from build123d import *

# Parameters (mm, degrees)
F2_SIZE = 1.5
F3_SIZE = 0.5


with BuildPart() as f1:
    # F0 (on Right) → F1 (revolve)
    with BuildSketch(Plane.YZ):
        Polygon((-3.7, 0), (-2, 0), (-2, 5), (-5.5, 5), (-5.5, 2.8), (-3.7, 2.8), align=None)
    revolve(axis=Axis((0, 0, 4.618393), (0, 0, 1)))

    # F2
    f2_edges = [f1.edges().sort_by_distance(p)[0] for p in [
        (0, 2, 5),
    ]]
    chamfer(f2_edges, length=F2_SIZE)

    # F3
    f3_edges = [f1.edges().sort_by_distance(p)[0] for p in [
        (0, 3.7, 0),
    ]]
    chamfer(f3_edges, length=F3_SIZE)


solid = f1.part
Can you work these out from the model? Positions are in its coordinate system, mm. A direction names the side the tool comes from. Coordinates: 2 decimals unless noted, no trailing zeros. Loops run counter-clockwise (first coordinate to the right, second up) from the corner with the lowest first, then second, coordinate; pieces in that order, holes last. Notation, with made-up numbers: (86, 33) - (102, 33) arc R23 ccw to (102, 67) - close; hole circle Ø7 at (44, 86). An arc over 180 degrees is marked (long way). Answer as a JSON object with one key per item and string values. Group by question number.
Item 1: On a 3-axis mill with a long thin cutter (end or side, diameter ignored), from which of +Z, -Z, +X, -X, +Y, -Y can I reach the whole of each face in a straight line? I mean faces 4 (the face through (-1, -4, 2.8)), 5 (the face through (0, 4, 5)). Say none if no direction works.
Item 2: If we section it at A-A (y = 0): List the corners of the cut face in (x, z) for me.
Item 3: If we mould it in two halves opening along Y, with no side actions, what happens to faces 1 (the face through (-1, -2, 0)), 2 (the face through (-2, 0, 2)), 3 (the face through (-5.37, 1.19, 3.88))? For each: released by +Y, released by -Y, zero draft, split by the parting line, or undercut.
Item 4: If we section it at C-C (z = 4.55): List the corners of the cut face in (x, y) for me.
Item 5: For pin 1 (5 mm diameter, centred on x = -2.5, y = -1.5, fed in from +Z); pin 2 (1 mm diameter, centred on x = -2, z = 4, fed in from -Y); pin 3 (3 mm diameter, centred on y = 0, z = 1, fed in from +X), each with a flat end and sliding along its axis, tell me the tip position at first contact or that it passes through.
Item 6: If we section it at D-D (z = 1.8): List the corners of the cut face in (x, y) for me, plus the area to 3 significant figures.
Item 7: If I drill on L1, parallel to X at y = 0, z = 2; L2, parallel to Z at x = 3.75, y = -1.75; L3, parallel to X at y = -1.25, z = 3.05, over which ranges is the centre line in solid material (lowest first)? Write a range as from..to.
Returned:
{
 "1": {"face 4": "-Z", "face 5": "+Z, +X, -X, +Y, -Y"},
 "2": {"outline": "(-5.5, 2.8) - (-3.7, 2.8) - (-3.7, 0.5) - (-3.2, 0) - (-2, 0) - (-2, 3.5) - (-3.5, 5) - (-5.5, 5) - close; (2, 0) - (3.2, 0) - (3.7, 0.5) - (3.7, 2.8) - (5.5, 2.8) - (5.5, 5) - (3.5, 5) - (2, 3.5) - close"},
 "3": {"face 1": "zero draft", "face 2": "undercut", "face 3": "split by the parting line"},
 "4": {"outline": "circle Ø11 at (0, 0); hole circle Ø6.1 at (0, 0)"},
 "5": {"pin 1": "stops at z = 5", "pin 2": "stops at y = -5.29", "pin 3": "stops at x = 3.7"},
 "6": {"outline": "circle Ø7.4 at (0, 0); hole circle Ø4 at (0, 0)", "area": "30.4 mm²"},
 "7": {"L1": "x = -3.7..-2, 2..3.7", "L2": "z = 2.8..5", "L3": "x = -5.36..-1.56, 1.56..5.36"}
}
